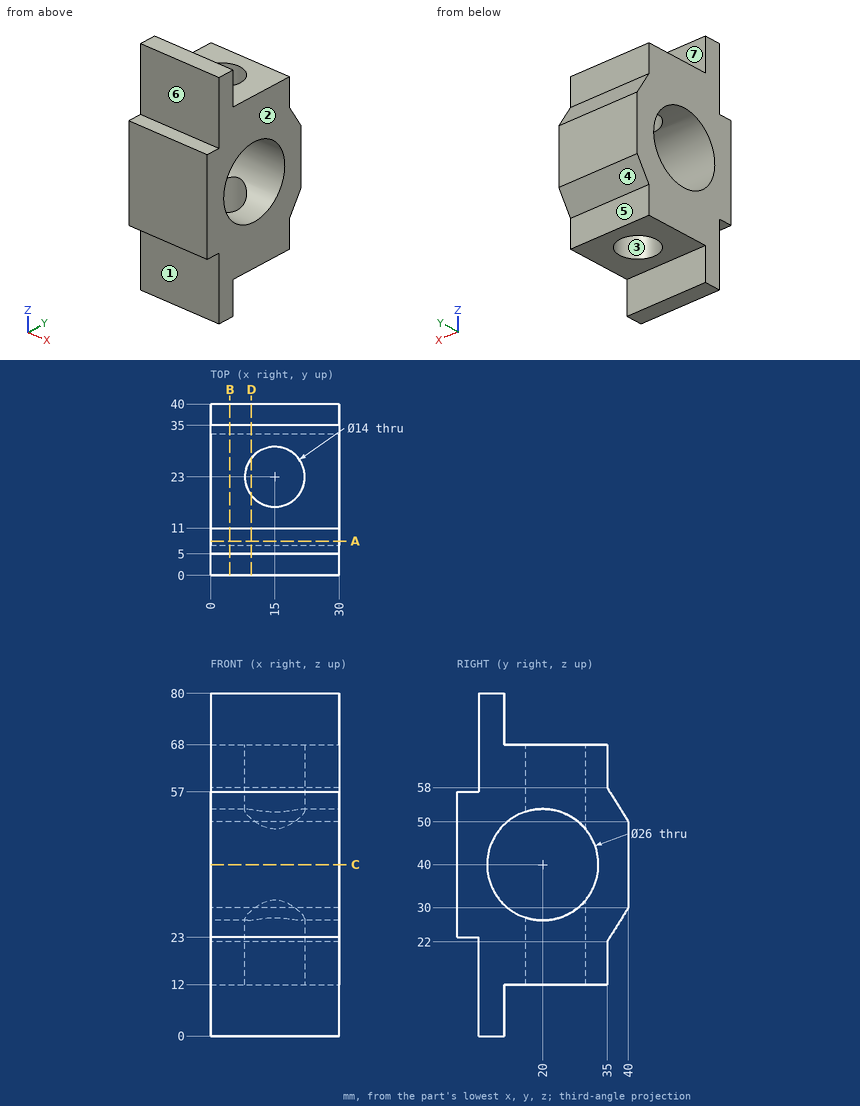
Design review of the part shown in the three views and the two pictorial views. Dimensions are in mm from the part's minimum x, y and z. A direction names the side the tool comes from. Round coordinates to 2 decimals unless told otherwise and drop trailing zeros. Loops run counter-clockwise (first coordinate to the right, second up) from the corner with the lowest first, then second, coordinate; pieces in that order, holes last.
1) Tool access review of the marked faces 5, 6 and 7: name each direction out of +Z, -Z, +X, -X, +Y, -Y from which nothing blocks a thin tool from reaching the whole face with its end or side.
Values follow:
face 5: -Z, +X, -X, +Y
face 6: +Z, +X, -X, -Y
face 7: +Z, +X, -X, +Y
2) Consider section D-D on x = 9.5. State the section outline as (y, z) points.
Values follow:
outline: (0, 23) - (5, 23) - (5, 0) - (11, 0) - (11, 12) - (18.67, 12) - (18.67, 27.07) arc R13 cw to (18.67, 52.93) - (18.67, 68) - (11, 68) - (11, 80) - (5, 80) - (5, 57) - (0, 57) - close; (27.33, 12) - (35, 12) - (35, 22) - (40, 30) - (40, 50) - (35, 58) - (35, 68) - (27.33, 68) - (27.33, 50.74) arc R13 cw to (27.33, 29.26) - close
3) Wall thickness on line 1 along X through (y, z) = (23, 24); line 2 along Y through (x, z) = (7, 40); line 3 along Y through (x, z) = (15, 19): over which ranges is each line inside the solid? List them lowest first.
Values follow:
line 1: x = 0 to 8, 22 to 30
line 2: y = 0 to 7, 33 to 40
line 3: y = 5 to 16, 30 to 35
4) Clearance check with flat-ended pins moving along their axes: P1, Ø3, axis at y = 27.5, z = 48, coming from the +X side; P2, Ø2, axis at x = 8.5, z = 65.5, coming from the -Y side; P3, Ø5, axis at x = 16, y = 27.5, coming from the -Z side; P4, Ø5, axis at x = 19.5, z = 17, coming from the +Y side. State where each tip first meets the part, or that it passes through.
Values follow:
P1: passes through
P2: stops at y = 5
P3: stops at z = 12
P4: stops at y = 35
5) Consider section A-A on y = 8. State the section outline as (x, z) points, then the cut area to 3 significant figures.
Values follow:
outline: (0, 0) - (30, 0) - (30, 35) - (0, 35) - close; (0, 45) - (30, 45) - (30, 80) - (0, 80) - close
area: 2,100 mm2
6) Consider section C-C on z = 40. State the section outline as (x, y) points.
Values follow:
outline: (0, 0) - (30, 0) - (30, 7) - (0, 7) - close; (0, 33) - (30, 33) - (30, 40) - (0, 40) - close
7) The part is to be moulded in two halves that separate along Y. For the marked faces 1, 2, 3 and 4, say which applies: pulls with the +Y half, pulls with the -Y half, needs draft (parallel to the pull), parting line crosses it, or undercut.
Values follow:
face 1: pulls with the -Y half
face 2: needs draft
face 3: undercut
face 4: pulls with the +Y half
8) Consider section B-B on x = 4.5. State the section outline as (y, z) points, then the cut area to 3 significant figures.
Values follow:
outline: (0, 23) - (5, 23) - (5, 0) - (11, 0) - (11, 12) - (35, 12) - (35, 22) - (40, 30) - (40, 50) - (35, 58) - (35, 68) - (11, 68) - (11, 80) - (5, 80) - (5, 57) - (0, 57) - close; hole circle Ø26 at (20, 40)
area: 1,600 mm2
